The listing builds one solid part. Answer for the finished solid, in the listing's coordinates (mm). Give positions to 0.01 mm unless a question says otherwise; leave off trailing zeros. Write each loop counter-clockwise with the first axis right and the second up, starting at its lowest first coordinate (ties: lowest second). Pieces come first, ordered by that corner, then holes. Notation, with made-up numbers: (42.5, -35) -> (69.5, -35) arc R30 ccw to (69.5, -9) -> close; hole circle Ø3 at (-34.75, -9.75). An arc over 180 degrees is marked (long way). One line per question, with ' | ' between items.
from build123d import *

# Parameters (mm, degrees)
SKETCH_1_W          = 35
SKETCH_1_H          = 9
EXTRUDE_1_DEPTH     = 5
SKETCH_2_R          = 0.725
SKETCH_2_R_2        = 1.25
SKETCH_2_R_3        = 0.4
CUT_EXTRUDE_1_DEPTH = 19.748333259


with BuildPart() as part:
    # 草图1 → 凸台-拉伸1 (new body)
    with BuildSketch(Plane(origin=(0, 0, 0), x_dir=(1, 0, 0), z_dir=(0, 1, 0))):
        Rectangle(SKETCH_1_W, SKETCH_1_H)
    extrude(amount=EXTRUDE_1_DEPTH)

    # 草图2 → 切除-拉伸1 (cut, through all)
    with BuildSketch(Plane(origin=(0, 5, 0), x_dir=(1, 0, 0), z_dir=(0, 1, 0))):
        with Locations(Location((-16, 3, 0), (0, 0, 270))):
            Circle(SKETCH_2_R)
        with Locations(Location((-13.090909091, 3, 0), (0, 0, 270))):
            Circle(SKETCH_2_R)
        with Locations(Location((-10.181818182, 3, 0), (0, 0, 270))):
            Circle(SKETCH_2_R)
        with Locations(Location((-7.272727273, 3, 0), (0, 0, 270))):
            Circle(SKETCH_2_R)
        with Locations(Location((-4.363636364, 3, 0), (0, 0, 270))):
            Circle(SKETCH_2_R)
        with Locations(Location((-1.454545455, 3, 0), (0, 0, 270))):
            Circle(SKETCH_2_R)
        with Locations(Location((1.454545455, 3, 0), (0, 0, 270))):
            Circle(SKETCH_2_R)
        with Locations(Location((4.363636364, 3, 0), (0, 0, 270))):
            Circle(SKETCH_2_R)
        with Locations(Location((7.272727273, 3, 0), (0, 0, 270))):
            Circle(SKETCH_2_R)
        with Locations(Location((10.181818182, 3, 0), (0, 0, 270))):
            Circle(SKETCH_2_R)
        with Locations(Location((13.090909091, 3, 0), (0, 0, 270))):
            Circle(SKETCH_2_R)
        with Locations(Location((16, 3, 0), (0, 0, 270))):
            Circle(SKETCH_2_R)
        with Locations(Location((-16, 0.4, 0), (0, 0, 270))):
            Circle(SKETCH_2_R_2)
        with Locations(Location((-13.090909091, 0.4, 0), (0, 0, 270))):
            Circle(SKETCH_2_R_2)
        with Locations(Location((-10.181818182, 0.4, 0), (0, 0, 270))):
            Circle(SKETCH_2_R_2)
        with Locations(Location((-7.272727273, 0.4, 0), (0, 0, 270))):
            Circle(SKETCH_2_R_2)
        with Locations(Location((-4.363636364, 0.4, 0), (0, 0, 270))):
            Circle(SKETCH_2_R_2)
        with Locations(Location((-1.454545455, 0.4, 0), (0, 0, 270))):
            Circle(SKETCH_2_R_2)
        with Locations(Location((1.454545455, 0.4, 0), (0, 0, 270))):
            Circle(SKETCH_2_R_2)
        with Locations(Location((4.363636364, 0.4, 0), (0, 0, 270))):
            Circle(SKETCH_2_R_2)
        with Locations(Location((7.272727273, 0.4, 0), (0, 0, 270))):
            Circle(SKETCH_2_R_2)
        with Locations(Location((10.181818182, 0.4, 0), (0, 0, 270))):
            Circle(SKETCH_2_R_2)
        with Locations(Location((13.090909091, 0.4, 0), (0, 0, 270))):
            Circle(SKETCH_2_R_2)
        with Locations(Location((16, 0.4, 0), (0, 0, 270))):
            Circle(SKETCH_2_R_2)
        with Locations(Location((-16, -2.2, 0), (0, 0, 270))):
            Circle(SKETCH_2_R)
        with Locations(Location((-13.090909091, -2.2, 0), (0, 0, 270))):
            Circle(SKETCH_2_R)
        with Locations(Location((-10.181818182, -2.2, 0), (0, 0, 270))):
            Circle(SKETCH_2_R)
        with Locations(Location((-7.272727273, -2.2, 0), (0, 0, 270))):
            Circle(SKETCH_2_R)
        with Locations(Location((-4.363636364, -2.2, 0), (0, 0, 270))):
            Circle(SKETCH_2_R)
        with Locations(Location((-1.454545455, -2.2, 0), (0, 0, 270))):
            Circle(SKETCH_2_R)
        with Locations(Location((1.454545455, -2.2, 0), (0, 0, 270))):
            Circle(SKETCH_2_R)
        with Locations(Location((4.363636364, -2.2, 0), (0, 0, 270))):
            Circle(SKETCH_2_R)
        with Locations(Location((7.272727273, -2.2, 0), (0, 0, 270))):
            Circle(SKETCH_2_R)
        with Locations(Location((10.181818182, -2.2, 0), (0, 0, 270))):
            Circle(SKETCH_2_R)
        with Locations(Location((13.090909091, -2.2, 0), (0, 0, 270))):
            Circle(SKETCH_2_R)
        with Locations(Location((16, -2.2, 0), (0, 0, 270))):
            Circle(SKETCH_2_R)
        with Locations(Location((-16.7, -3.9, 0), (0, 0, 270))):
            Circle(SKETCH_2_R_3)
        with Locations(Location((-14.939473684, -3.9, 0), (0, 0, 270))):
            Circle(SKETCH_2_R_3)
        with Locations(Location((-13.178947368, -3.9, 0), (0, 0, 270))):
            Circle(SKETCH_2_R_3)
        with Locations(Location((-11.418421053, -3.9, 0), (0, 0, 270))):
            Circle(SKETCH_2_R_3)
        with Locations(Location((-9.657894737, -3.9, 0), (0, 0, 270))):
            Circle(SKETCH_2_R_3)
        with Locations(Location((-7.897368421, -3.9, 0), (0, 0, 270))):
            Circle(SKETCH_2_R_3)
        with Locations(Location((-6.136842105, -3.9, 0), (0, 0, 270))):
            Circle(SKETCH_2_R_3)
        with Locations(Location((-4.376315789, -3.9, 0), (0, 0, 270))):
            Circle(SKETCH_2_R_3)
        with Locations(Location((-2.615789474, -3.9, 0), (0, 0, 270))):
            Circle(SKETCH_2_R_3)
        with Locations(Location((-0.855263158, -3.9, 0), (0, 0, 270))):
            Circle(SKETCH_2_R_3)
        with Locations(Location((0.905263158, -3.9, 0), (0, 0, 270))):
            Circle(SKETCH_2_R_3)
        with Locations(Location((2.665789474, -3.9, 0), (0, 0, 270))):
            Circle(SKETCH_2_R_3)
        with Locations(Location((4.426315789, -3.9, 0), (0, 0, 270))):
            Circle(SKETCH_2_R_3)
        with Locations(Location((6.186842105, -3.9, 0), (0, 0, 270))):
            Circle(SKETCH_2_R_3)
        with Locations(Location((7.947368421, -3.9, 0), (0, 0, 270))):
            Circle(SKETCH_2_R_3)
        with Locations(Location((9.707894737, -3.9, 0), (0, 0, 270))):
            Circle(SKETCH_2_R_3)
        with Locations(Location((11.468421053, -3.9, 0), (0, 0, 270))):
            Circle(SKETCH_2_R_3)
        with Locations(Location((13.228947368, -3.9, 0), (0, 0, 270))):
            Circle(SKETCH_2_R_3)
        with Locations(Location((14.989473684, -3.9, 0), (0, 0, 270))):
            Circle(SKETCH_2_R_3)
        with Locations(Location((16.75, -3.9, 0), (0, 0, 270))):
            Circle(SKETCH_2_R_3)
    extrude(amount=-CUT_EXTRUDE_1_DEPTH, mode=Mode.SUBTRACT)


solid = part.part
Item 1: Find section B-B (z = -0.4). Count the separate pieces of the cut face and the enclosed holes in it, then the cut area to 3 significant figures.
Answers below:
separate pieces: 13 | enclosed holes: 0 | area: 25.0 mm²
Item 2: Consider line 1 (Z direction, x = -1, y = 0.7); line 2 (Z direction, x = -15, y = 2.3); line 3 (Z direction, x = -5, y = 2.8). Determine where each line is inside the solid, lowest interval first. Write a range as [from, to].
Answers below:
line 1: [-4.5, -3.56], [-2.44, -1.56], [0.76, 1.64], [2.76, 3.53], [4.27, 4.5] | line 2: [-4.5, -1.15], [0.35, 3.5], [4.3, 4.5] | line 3: [-4.5, -3.35], [-2.65, -1.48], [0.68, 1.85], [2.55, 4.5]
Item 3: A flat-ended cylindrical pin translates along its axis: pin 1 (1.2 mm diameter, centred on x = 1.45, z = -3, fed in from +Y). Find the tip coordinate at first contact, or state that the pin passes through.
Answers below:
pin 1: through
Item 4: Find section A-A (x = -16). Write down the section's boundary in (y, z) (3 decimals), then the cut area to 3 significant figures.
Answers below:
outline: (0, -4.5) -> (5, -4.5) -> (5, -3.725) -> (0, -3.725) -> close; (0, -2.275) -> (5, -2.275) -> (5, -1.65) -> (0, -1.65) -> close; (0, 0.85) -> (5, 0.85) -> (5, 1.475) -> (0, 1.475) -> close; (0, 2.925) -> (5, 2.925) -> (5, 4.5) -> (0, 4.5) -> close | area: 18.0 mm²
Item 5: Determine the mould class of faces 1 (the face through (0, 2, -4.5)), 2 (the face through (-12.842, 2.535, 4.115)) for opening direction X: pulls with the +X half, pulls with the -X half, needs draft (parallel to the pull), parting line crosses it, or undercut.
Answers below:
face 1: needs draft | face 2: undercut
